The model under review builds one solid part; all positions refer to its coordinate system, in mm. Face numbers are marked on the shaded views. A direction names the side the tool comes from. Coordinates: 2 decimals unless noted, no trailing zeros. Write each loop counter-clockwise with the first axis right and the second up, starting at its lowest first coordinate (ties: lowest second). Pieces come first, ordered by that corner, then holes. Notation, with made-up numbers: (5, -33) - (11, -33) arc R20 ccw to (11, 0) - close; hole circle Ø4 at (-13, 36). An arc over 180 degrees is marked (long way). Put each result on its own line as item: value. Start each with the question number.
Item 1: For pin 1 (6 mm diameter, centred on x = 5, y = -9.5, fed in from +Z); pin 2 (1.5 mm diameter, centred on x = -2, y = -8, fed in from +Z); pin 3 (3.5 mm diameter, centred on x = 0, z = 11.95, fed in from +Y), all flat-tipped, find the tip position at first contact; note any pin that passes through.
Item 2: Consider section A-A on x = 0. Give the boundary of the cut face in (y, z).
Item 3: Consider section B-B on z = 6.5. Give the boundary of the cut face in (x, y), then the cut area to 3 significant figures.
Item 4: Machinability: for the marked faces 1 and 2, which of the approach directions +Z, -Z, +X, -X, +Y, -Y give a long, thin tool a straight path to every point of the face, cutting with its end or side? Answer none if there is none.
Item 5: Consider section D-D on y = -2. Give the boundary of the cut face in (x, z).
Item 6: Mouldability with a two-part tool opening along Z and no side actions: class the marked faces 3, 4 and 5 as pulls with the +Z half, pulls with the -Z half, needs draft (parallel to the pull), parting line crosses it, or undercut.
Item 7: To check wall thickness, follow L1, parallel to Y at x = -2.5, z = 8.5; L2, parallel to Z at x = 0, y = -13.7; L3, parallel to Z at x = 1.75, y = -6.25. State the ranges of each line that lie inside material, in increasing order. Write a range as [from, to].
Item 8: Consider section C-C on y = -12.25. Give the boundary of the cut face in (x, z).
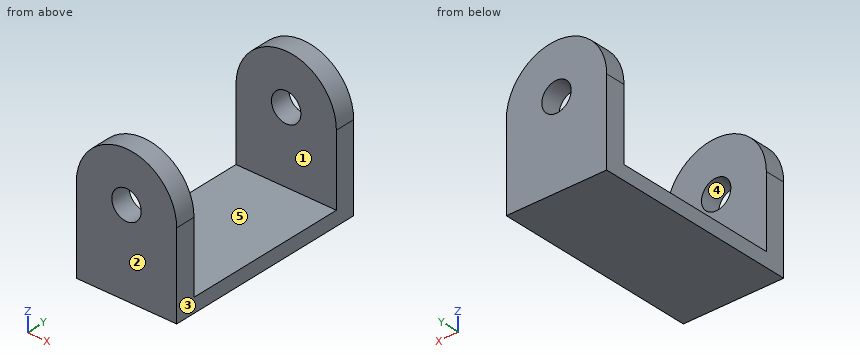
```python
from build123d import *

# Parameters (mm, degrees)
F1_R     = 2.05
F2_DEPTH = 2.8
F3_W     = 14
F3_H     = 2
F4_DEPTH = 11.5


with BuildPart() as f2:
    # F1 (on offset) → F2 (new body)
    with BuildSketch(Plane.XZ.offset(11.5)):
        with BuildLine():
            Line((-7, 11.95), (-7, 0))
            Line((-7, 0), (7, 0))
            Line((7, 0), (7, 11.95))
            ThreePointArc((7, 11.95), (0, 18.95), (-7, 11.95))
        make_face()
        with Locations((0, 11.95)):
            Circle(F1_R, mode=Mode.SUBTRACT)
    extrude(amount=F2_DEPTH)

    # F3 (on face) → F4 (join, through all)
    with BuildSketch(Plane(origin=(0, -11.5, 0), x_dir=(-1, 0, 0), z_dir=(0, 1, 0))):
        with Locations((0, 1)):
            Rectangle(F3_W, F3_H)
    extrude(amount=F4_DEPTH)

    # F5: F2 across plane


with BuildPart() as f2_1:
    add(f2.part)
    add(f2.part.mirror(Plane.XZ))


solid = f2_1.part
```
Report:
1. pin 1: z = 18.38
1. pin 2: z = 2
1. pin 3: through
2. outline: (-14.3, 0) - (14.3, 0) - (14.3, 9.9) - (11.5, 9.9) - (11.5, 2) - (-11.5, 2) - (-11.5, 9.9) - (-14.3, 9.9) - close; (-14.3, 14) - (-11.5, 14) - (-11.5, 18.95) - (-14.3, 18.95) - close; (11.5, 14) - (14.3, 14) - (14.3, 18.95) - (11.5, 18.95) - close
3. outline: (-7, -14.3) - (7, -14.3) - (7, -11.5) - (-7, -11.5) - close; (-7, 11.5) - (7, 11.5) - (7, 14.3) - (-7, 14.3) - close
3. area: 78.4 mm²
4. face 1: +Z, +X, -X
4. face 2: +Z, -Z, +X, -X, -Y
5. outline: (-7, 0) - (7, 0) - (7, 2) - (-7, 2) - close
6. face 3: needs draft
6. face 4: undercut
6. face 5: pulls with the +Z half
7. L1: [-14.3, -11.5], [11.5, 14.3]
7. L2: [0, 9.9], [14, 18.95]
7. L3: [0, 2]
8. outline: (-7, 0) - (7, 0) - (7, 11.95) arc R7 ccw to (-7, 11.95) - close; hole circle Ø4.1 at (0, 11.95)
